For this review, take the finished solid that the model builds, in its own axes (mm). Give positions to 0.01 mm unless a question says otherwise; leave off trailing zeros. Loops run counter-clockwise (first coordinate to the right, second up) from the corner with the lowest first, then second, coordinate; pieces in that order, holes last.
```python
from build123d import *

# Parameters (mm, degrees)
ESQUISSE1_R      = 1.9
EXTRUSION1_DEPTH = 2
D_POUILLE2_ANGLE = 2
CHANFREIN1_SIZE  = 1
CHANFREIN1_SIZE2 = 1.056596466
CHANFREIN2_SIZE  = 1
CHANFREIN2_SIZE2 = 1.056596466
CHANFREIN4_SIZE  = 1
CHANFREIN4_SIZE2 = 0.951621439
CHANFREIN5_SIZE  = 1
CHANFREIN5_SIZE2 = 0.951621439


with BuildPart() as part:
    # Esquisse1 → Extrusion1 (new body)
    with BuildSketch(Plane.XY):
        Polygon((32.89280914, 0), (32.89280914, 45), (-187.10719086, 33.5), (-187.10719086, 0), align=None)
        with Locations((-182.10719086, 28)):
            Circle(ESQUISSE1_R, mode=Mode.SUBTRACT)
        with Locations((27.89280914, 40)):
            Circle(ESQUISSE1_R, mode=Mode.SUBTRACT)
    extrude(amount=EXTRUSION1_DEPTH)

    # Dépouille2
    d_pouille2_faces = [part.faces().sort_by_distance(p)[0] for p in [
        (-71.721493892, 19.727903034, 0),
    ]]
    draft(d_pouille2_faces, Plane(origin=(32.89280914, 0, 2), x_dir=(-1, 0, 0), z_dir=(0, -1, 0)), D_POUILLE2_ANGLE)

    # Symétrie1: part across plane


with BuildPart() as part_1:
    add(part.part)
    add(part.part.mirror(Plane(origin=(32.89280914, 0, 2), x_dir=(0, 0, 1), z_dir=(0, 1, 0))))

    # Chanfrein1
    chanfrein1_edges = [part_1.edges().sort_by_distance(p)[0] for p in [
        (-187.10719086, 33.5, 0.415077111),
    ]]
    chanfrein1_side = [part_1.faces().sort_by_distance(p)[0] for p in [
        (-74.922898918, 39.364178897, 0.312686291),
    ]]
    chamfer(chanfrein1_edges, length=CHANFREIN1_SIZE, length2=CHANFREIN1_SIZE2, reference=chanfrein1_side[0])

    # Chanfrein2
    chanfrein2_edges = [part_1.edges().sort_by_distance(p)[0] for p in [
        (-187.10719086, -33.5, 0.415077111),
    ]]
    chanfrein2_side = [part_1.faces().sort_by_distance(p)[0] for p in [
        (-187.10719086, -0.646362154, 0.690599114),
    ]]
    chamfer(chanfrein2_edges, length=CHANFREIN2_SIZE, length2=CHANFREIN2_SIZE2, reference=chanfrein2_side[0])

    # Chanfrein4
    chanfrein4_edges = [part_1.edges().sort_by_distance(p)[0] for p in [
        (32.89280914, -45, 0.214282686),
    ]]
    chanfrein4_side = [part_1.faces().sort_by_distance(p)[0] for p in [
        (-74.416841112, -39.390631919, 0.312224411),
    ]]
    chamfer(chanfrein4_edges, length=CHANFREIN4_SIZE, length2=CHANFREIN4_SIZE2, reference=chanfrein4_side[0])

    # Chanfrein5
    chanfrein5_edges = [part_1.edges().sort_by_distance(p)[0] for p in [
        (32.89280914, 45, 0.214282686),
    ]]
    chanfrein5_side = [part_1.faces().sort_by_distance(p)[0] for p in [
        (32.89280914, 0.608982965, 0.574960444),
    ]]
    chamfer(chanfrein5_edges, length=CHANFREIN5_SIZE, length2=CHANFREIN5_SIZE2, reference=chanfrein5_side[0])


solid = part_1.part
```
Q1. For pin 1 Ø3 at (x, y) = (27.89, -40) entering from +Z; pin 2 Ø10 at (x, y) = (-80, 22) entering from -Z; pin 3 Ø5 at (x, y) = (-182.11, 28) entering from -Z, all flat-tipped, find the tip position at first contact; note any pin that passes through.
Answers:
pin 1: passes through
pin 2: stops at z = -0.94
pin 3: stops at z = -1.07
Q2. Mouldability with a two-part tool opening along Y and no side actions: class faces 1 (the cylindrical face through (-184.005, -28.084, 0.45)), 2 (the flat face through (-79, -1, 2)), 3 (the flat face through (-75.55, -39.33, 0.19)) as +Y half, -Y half, draft (parallel to the pull), parting line (faces both ways), or undercut.
Answers:
face 1: undercut
face 2: draft
face 3: -Y half
Q3. Consider section B-B on x = -148. Give the boundary of the cut face in (y, z).
Answers:
outline: (-35.54, -1.24) - (0, 0) - (35.54, -1.24) - (35.54, 2) - (-35.54, 2) - close
Q4. Consider section A-A on z = 0.55. Give the boundary of the cut face in (x, y), plus the area to 3 significant figures.
Answers:
outline: (-187.11, -32.5) - (-186.05, -33.56) - (31.89, -44.95) - (32.89, -44.05) - (32.89, 44) - (31.94, 44.95) - (-186.11, 33.55) - (-187.11, 32.44) - close; hole circle Ø3.8 at (-182.11, -28); hole circle Ø3.8 at (-182.11, 28); hole circle Ø3.8 at (27.89, -40); hole circle Ø3.8 at (27.89, 40)
area: 17,200 mm2
Q5. Consider section C-C on y = 3. Give the boundary of the cut face in (x, z), plus the area to 3 significant figures.
Answers:
outline: (-187.11, -0.1) - (32.89, -0.1) - (32.89, 2) - (-187.11, 2) - close
area: 463 mm2
Q6. For probe 1 along X at (y, z) = (-28, -0.05); probe 2 along Z at (x, y) = (-51, -33); probe 3 along Z at (x, y) = (-158.5, -30.5), list the stretches that pass through material, from the lowest coordinate up.
Answers:
probe 1: x = -187.11 to -184.01, -180.21 to 32.89
probe 2: z = -1.15 to 2
probe 3: z = -1.07 to 2
Q7. Consider section D-D on x = -116. Give the boundary of the cut face in (y, z), plus the area to 3 significant figures.
Answers:
outline: (-37.22, -1.3) - (0, 0) - (37.22, -1.3) - (37.22, 2) - (-37.22, 2) - close
area: 197 mm2
